```python
from build123d import *

# Parameters (mm, degrees)
CYLINDER099_R               = 3
CYLINDER099_DEPTH           = 3
CYLINDER098_R               = 5
CYLINDER098_DEPTH           = 3
CYLINDER090_R               = 1.2
CYLINDER090_DEPTH           = 13
CYLINDER091_R               = 1
CYLINDER091_DEPTH           = 12
CYLINDER091_ROLL_ANGLE      = 89.999919
CYLINDER091_PITCH_ANGLE     = -3.6e-05
CYLINDER091_PLACEMENT_ANGLE = 179.999964
CYLINDER069_R               = 2.2
CYLINDER069_DEPTH           = 12
CYLINDER069_ROLL_ANGLE      = 89.999919
CYLINDER069_PITCH_ANGLE     = -3.6e-05
CYLINDER069_PLACEMENT_ANGLE = 179.999964
CYLINDER068_R               = 1.2
CYLINDER068_DEPTH           = 12
CYLINDER068_ROLL_ANGLE      = 89.999919
CYLINDER068_PITCH_ANGLE     = -3.6e-05
CYLINDER068_PLACEMENT_ANGLE = 179.999964
BOX406016_W                 = 49
BOX406016_H                 = 2
BOX406016_DEPTH             = 32
BOX406008016_W              = 9
BOX406008016_H              = 12
BOX406008016_DEPTH          = 15
BOX406017_W                 = 16
BOX406017_H                 = 10.5
BOX406017_DEPTH             = 28
CYLINDER067_R               = 7
CYLINDER067_DEPTH           = 26
COMMON004_PLACEMENT_ANGLE   = 90
BOX406008015_W              = 15
BOX406008015_H              = 31
BOX406008015_DEPTH          = 15
BOX406008017_W              = 15
BOX406008017_H              = 4
BOX406008017_DEPTH          = 24
CYLINDER096_R               = 1.7
CYLINDER096_DEPTH           = 21
BOX_W                       = 15
BOX_H                       = 3
BOX_DEPTH                   = 8
CYLINDER097_R               = 1.7
CYLINDER097_DEPTH           = 21
BOX406008018_W              = 15
BOX406008018_H              = 3
BOX406008018_DEPTH          = 8
CHAMFER005_SIZE             = 1
CYLINDER093_R               = 1.7
CYLINDER093_DEPTH           = 21
CYLINDER092_R               = 1.7
CYLINDER092_DEPTH           = 21
BOX406008014_W              = 15
BOX406008014_H              = 3
BOX406008014_DEPTH          = 63
CHAMFER006_SIZE             = 1
CHAMFER007_SIZE             = 6.5
CHAMFER009_SIZE             = 0.5
CHAMFER010_SIZE             = 0.5


with BuildPart() as cylinder099:
    # Cylinder099 → Cylinder099 (new body)
    with BuildSketch(Plane(origin=(-9, -9, 36), x_dir=(1, 0, 0), z_dir=(0, 0, 1))):
        Circle(CYLINDER099_R)
    extrude(amount=CYLINDER099_DEPTH)


with BuildPart() as cut081:
    # Cylinder098 → Cylinder098 (new body)
    with BuildSketch(Plane(origin=(-9, -9, 36), x_dir=(1, 0, 0), z_dir=(0, 0, 1))):
        Circle(CYLINDER098_R)
    extrude(amount=CYLINDER098_DEPTH)

    # Cut081: cut Cylinder099
    add(cylinder099.part, mode=Mode.SUBTRACT)


with BuildPart() as cylinder084:
    # Cylinder090 → Cylinder090 (new body)
    with BuildSketch(Plane(origin=(0, 16, 35.8), x_dir=(1, 0, 0), z_dir=(0, -1, 0))):
        Circle(CYLINDER090_R)
    extrude(amount=CYLINDER090_DEPTH)


with BuildPart() as cylinder091:
    # Cylinder091 → Cylinder091 (new body)
    with BuildSketch(Plane.XY):
        Circle(CYLINDER091_R)
    extrude(amount=CYLINDER091_DEPTH)


with BuildPart() as cylinder091_1:
    # Cylinder091 roll: moved
    add(cylinder091.part.rotate(Axis((0, 0, 0), (1, 0, 0)), CYLINDER091_ROLL_ANGLE))


with BuildPart() as cylinder091_2:
    # Cylinder091 pitch: moved
    add(cylinder091_1.part.rotate(Axis((0, 0, 0), (0, 1, 0)), CYLINDER091_PITCH_ANGLE))


with BuildPart() as cylinder091_3:
    # Cylinder091 placement: moved
    add(cylinder091_2.part.moved(Location((11.75, -12, 42.5))).rotate(Axis((11.75, -12, 42.5), (0, 0, 1)), CYLINDER091_PLACEMENT_ANGLE))


with BuildPart() as cylinder069:
    # Cylinder069 → Cylinder069 (new body)
    with BuildSketch(Plane.XY):
        Circle(CYLINDER069_R)
    extrude(amount=CYLINDER069_DEPTH)


with BuildPart() as cylinder069_1:
    # Cylinder069 roll: moved
    add(cylinder069.part.rotate(Axis((0, 0, 0), (1, 0, 0)), CYLINDER069_ROLL_ANGLE))


with BuildPart() as cylinder069_2:
    # Cylinder069 pitch: moved
    add(cylinder069_1.part.rotate(Axis((0, 0, 0), (0, 1, 0)), CYLINDER069_PITCH_ANGLE))


with BuildPart() as cylinder069_3:
    # Cylinder069 placement: moved
    add(cylinder069_2.part.moved(Location((11.75, 3, 42.5))).rotate(Axis((11.75, 3, 42.5), (0, 0, 1)), CYLINDER069_PLACEMENT_ANGLE))


with BuildPart() as fusion103077013004017011:
    # Cylinder068 → Cylinder068 (new body)
    with BuildSketch(Plane.XY):
        Circle(CYLINDER068_R)
    extrude(amount=CYLINDER068_DEPTH)


with BuildPart() as fusion103077013004017011_1:
    # Cylinder068 roll: moved
    add(fusion103077013004017011.part.rotate(Axis((0, 0, 0), (1, 0, 0)), CYLINDER068_ROLL_ANGLE))


with BuildPart() as fusion103077013004017011_2:
    # Cylinder068 pitch: moved
    add(fusion103077013004017011_1.part.rotate(Axis((0, 0, 0), (0, 1, 0)), CYLINDER068_PITCH_ANGLE))


with BuildPart() as fusion103077013004017011_3:
    # Cylinder068 placement: moved
    add(fusion103077013004017011_2.part.moved(Location((11.75, 0, 42.5))).rotate(Axis((11.75, 0, 42.5), (0, 0, 1)), CYLINDER068_PLACEMENT_ANGLE))

    # Fusion103077013: union Cylinder069
    add(cylinder069_3.part)

    # Fusion103077013004017011: union Cylinder091
    add(cylinder091_3.part)


with BuildPart() as clamp_slot:
    # Box406016 → Box406016 (new body)
    with BuildSketch(Plane(origin=(48.48, 1, 22), x_dir=(-1, 0, 0), z_dir=(0, 0, 1))):
        with Locations((24.5, 1)):
            Rectangle(BOX406016_W, BOX406016_H)
    extrude(amount=BOX406016_DEPTH)


with BuildPart() as cube351:
    # Box406008016 → Box406008016 (new body)
    with BuildSketch(Plane(origin=(7, -6, 35), x_dir=(1, 0, 0), z_dir=(0, 0, 1))):
        with Locations((4.5, 6)):
            Rectangle(BOX406008016_W, BOX406008016_H)
    extrude(amount=BOX406008016_DEPTH)


with BuildPart() as gearbox001:
    # Box406017 → Box406017 (new body)
    with BuildSketch(Plane(origin=(-8, -5.25, 18), x_dir=(1, 0, 0), z_dir=(0, 0, 1))):
        with Locations((8, 5.25)):
            Rectangle(BOX406017_W, BOX406017_H)
    extrude(amount=BOX406017_DEPTH)


with BuildPart() as motor_hole:
    # Cylinder067 → Cylinder067 (new body)
    with BuildSketch(Plane.XY.offset(20)):
        Circle(CYLINDER067_R)
    extrude(amount=CYLINDER067_DEPTH)

    # Common004: intersect gearbox001
    add(gearbox001.part, mode=Mode.INTERSECT)


with BuildPart() as motor_hole_1:
    # Common004 placement: moved
    add(motor_hole.part.moved(Location((0, 0, 5))).rotate(Axis((0, 0, 5), (0, 0, 1)), COMMON004_PLACEMENT_ANGLE))


with BuildPart() as cut075:
    # Box406008015 → Box406008015 (new body)
    with BuildSketch(Plane(origin=(-7.5, -22, 35), x_dir=(1, 0, 0), z_dir=(0, 0, 1))):
        with Locations((7.5, 15.5)):
            Rectangle(BOX406008015_W, BOX406008015_H)
    extrude(amount=BOX406008015_DEPTH)

    # Cut073: cut motor-hole
    add(motor_hole_1.part, mode=Mode.SUBTRACT)

    # Fusion103077013004017010: union Cube351
    add(cube351.part)

    # Cut074: cut clamp-slot
    add(clamp_slot.part, mode=Mode.SUBTRACT)

    # Cut075: cut Fusion103077013004017011
    add(fusion103077013004017011_3.part, mode=Mode.SUBTRACT)


with BuildPart() as cut082:
    # Box406008017 → Box406008017 (new body)
    with BuildSketch(Plane(origin=(-7.5, 7, 26), x_dir=(1, 0, 0), z_dir=(0, 0, 1))):
        with Locations((7.5, 2)):
            Rectangle(BOX406008017_W, BOX406008017_H)
    extrude(amount=BOX406008017_DEPTH)

    # Fusion103077013004017012: union Cut075
    add(cut075.part)

    # Cut076: cut Cylinder084
    add(cylinder084.part, mode=Mode.SUBTRACT)


with BuildPart() as cut082_1:
    # Cut076 placement: moved
    add(cut082.part.moved(Location((0, 0, -5))))

    # Cut082: cut Cut081
    add(cut081.part, mode=Mode.SUBTRACT)


with BuildPart() as cylinder096:
    # Cylinder096 → Cylinder096 (new body)
    with BuildSketch(Plane(origin=(0, -13, 49), x_dir=(1, 0, 0), z_dir=(0, -1, 0))):
        Circle(CYLINDER096_R)
    extrude(amount=CYLINDER096_DEPTH)


with BuildPart() as cut080:
    # Box → Box (new body)
    with BuildSketch(Plane(origin=(-7.5, -25, 45), x_dir=(1, 0, 0), z_dir=(0, 0, 1))):
        with Locations((7.5, 1.5)):
            Rectangle(BOX_W, BOX_H)
    extrude(amount=BOX_DEPTH)

    # Cut080: cut Cylinder096
    add(cylinder096.part, mode=Mode.SUBTRACT)


with BuildPart() as cylinder097:
    # Cylinder097 → Cylinder097 (new body)
    with BuildSketch(Plane(origin=(0, -13, -22), x_dir=(1, 0, 0), z_dir=(0, -1, 0))):
        Circle(CYLINDER097_R)
    extrude(amount=CYLINDER097_DEPTH)


with BuildPart() as chamfer005:
    # Box406008018 → Box406008018 (new body)
    with BuildSketch(Plane(origin=(-7.5, -25, -26), x_dir=(1, 0, 0), z_dir=(0, 0, 1))):
        with Locations((7.5, 1.5)):
            Rectangle(BOX406008018_W, BOX406008018_H)
    extrude(amount=BOX406008018_DEPTH)

    # Cut079: cut Cylinder097
    add(cylinder097.part, mode=Mode.SUBTRACT)

    # Fusion103077013004017015: union Cut080
    add(cut080.part)

    # Chamfer005
    chamfer005_edges = [chamfer005.edges().sort_by_distance(p)[0] for p in [
        (-1.7, -22, -22),
        (-1.7, -22, 49),
    ]]
    chamfer(chamfer005_edges, length=CHAMFER005_SIZE)


with BuildPart() as cylinder093:
    # Cylinder093 → Cylinder093 (new body)
    with BuildSketch(Plane(origin=(3, -13, -4), x_dir=(1, 0, 0), z_dir=(0, -1, 0))):
        Circle(CYLINDER093_R)
    extrude(amount=CYLINDER093_DEPTH)


with BuildPart() as fusion103077013004017013:
    # Cylinder092 → Cylinder092 (new body)
    with BuildSketch(Plane(origin=(-3, -13, -14), x_dir=(1, 0, 0), z_dir=(0, -1, 0))):
        Circle(CYLINDER092_R)
    extrude(amount=CYLINDER092_DEPTH)

    # Fusion103077013004017013: union Cylinder093
    add(cylinder093.part)


with BuildPart() as chamfer010:
    # Box406008014 → Box406008014 (new body)
    with BuildSketch(Plane(origin=(-7.5, -25, -18), x_dir=(1, 0, 0), z_dir=(0, 0, 1))):
        with Locations((7.5, 1.5)):
            Rectangle(BOX406008014_W, BOX406008014_H)
    extrude(amount=BOX406008014_DEPTH)

    # Cut077: cut Fusion103077013004017013
    add(fusion103077013004017013.part, mode=Mode.SUBTRACT)

    # Chamfer006
    chamfer006_edges = [chamfer010.edges().sort_by_distance(p)[0] for p in [
        (-4.7, -25, -14),
        (1.3, -25, -4),
    ]]
    chamfer(chamfer006_edges, length=CHAMFER006_SIZE)

    # Fusion103077013004017016: union Chamfer005
    add(chamfer005.part)

    # Chamfer007
    chamfer007_edges = [chamfer010.edges().sort_by_distance(p)[0] for p in [
        (-7.5, -23.5, -26),
        (7.5, -23.5, -26),
        (7.5, -23.5, 53),
        (-7.5, -23.5, 53),
    ]]
    chamfer(chamfer007_edges, length=CHAMFER007_SIZE)

    # Fusion103077013004017017: union Cut082
    add(cut082_1.part)

    # Chamfer009
    chamfer009_edges = [chamfer010.edges().sort_by_distance(p)[0] for p in [
        (-4.7, -22, -14),
        (1.3, -22, -4),
    ]]
    chamfer(chamfer009_edges, length=CHAMFER009_SIZE)

    # Chamfer010
    chamfer010_edges = [chamfer010.edges().sort_by_distance(p)[0] for p in [
        (-1.7, -25, -22),
        (-1.7, -25, 49),
    ]]
    chamfer(chamfer010_edges, length=CHAMFER010_SIZE)


solid = chamfer010.part
```
The model under review builds one solid part; all positions refer to its coordinate system, in mm. A direction names the side the tool comes from. Coordinates: 2 decimals unless noted, no trailing zeros. Write each loop counter-clockwise with the first axis right and the second up, starting at its lowest first coordinate (ties: lowest second). Pieces come first, ordered by that corner, then holes. Notation, with made-up numbers: (7.25, 33) -> (59.25, 33) arc R14 ccw to (59.25, 42) -> close; hole circle Ø9 at (21.25, 53). An arc over 180 degrees is marked (long way). One line per item, written item: value. Start each with the question number.
Q1. Add section A-A, the plane z = -14. Give the boundary of the cut face in (x, y), then the cut area to 4 significant figures.
Q2. Clearance check with flat-ended pins moving along their axes: P1, Ø2.5, axis at x = 0, z = 49, coming from the +Y side; P2, Ø1.8, axis at x = -6.5, y = -7.5, coming from the +Z side; P3, Ø4, axis at y = -19.5, z = 44, coming from the +X side; P4, Ø6.5, axis at x = 5.5, y = 3.5, coming from the -Z side. State where each tip first meets the part, or that it passes through.
Q3. To check wall thickness, follow probe 1 along Z at (x, y) = (0, -24.05); probe 2 along X at (y, z) = (-3.45, 37.5); probe 3 along Z at (x, y) = (11.75, 5.15). State the ranges of each line that lie inside material, in increasing order.
Q4. The part is to be moulded in two halves that separate along Y. For faces 1 (the face through (-0.221, -23.74, -20.314)), 2 (the face through (0, -22, 46)), 3 (the face through (10, 4, 30)), 4 (the face through (0, 7, 25)), say which applies: +Y half, -Y half, draft (parallel to the pull), parting line (faces both ways), or undercut.
Q5. Add section D-D, the plane y = -12.5. Give the boundary of the cut face in (x, z).
Q6. Add section C-C, the plane z = 49. Give the boundary of the cut face in (x, y), then the cut area to 4 significant figures.
Q7. Add section B-B, the plane y = 2. Count the separate pieces of the cut face and the enclosed holes in it, then the cut area to 3 significant figures.
Q8. For faces 5 (the face through (5.25, -3, 37)), 6 (the face through (10, -1, 37)), 7 (the face through (0, -23, 53)), 8 (the face through (-0.26, 8.98, 29.63)), 9 (the face through (7.5, 8, 33)), list the 3-axis set-ups (+Z, -Z, +X, -X, +Y, -Y) from which the entire face can be reached by the end or side of a thin tool; tool diameter is ignored.
Response:
1. outline: (-7.5, -25) -> (-5.7, -25) -> (-4.7, -24) -> (-4.7, -22.5) -> (-5.2, -22) -> (-7.5, -22) -> close; (-1.3, -24) -> (-0.3, -25) -> (7.5, -25) -> (7.5, -22) -> (-0.8, -22) -> (-1.3, -22.5) -> close
1. area: 33.55 mm²
2. P1: through
2. P2: z = 45
2. P3: x = 7.5
2. P4: z = 30
3. probe 1: -26 to -23.7, -20.3 to 47.3, 50.7 to 53
3. probe 2: -7.5 to -5.25, 5.25 to 10.75, 12.75 to 16
3. probe 3: 30 to 35.3, 39.7 to 45
4. face 1: draft
4. face 2: +Y half
4. face 3: undercut
4. face 4: undercut
5. outline: (-7.5, 30) -> (7.5, 30) -> (7.5, 45) -> (-7.5, 45) -> (-7.5, 39) -> (-5.43, 39) -> (-5.43, 36) -> (-7.5, 36) -> close
6. outline: (-5, -25) -> (-2.2, -25) -> (-1.7, -24.5) -> (-1.7, -23) -> (-2.7, -22) -> (-5, -22) -> close; (1.7, -24.5) -> (2.2, -25) -> (5, -25) -> (5, -22) -> (2.7, -22) -> (1.7, -23) -> close
6. area: 18.55 mm²
7. separate pieces: 2
7. enclosed holes: 1
7. area: 190 mm²
8. face 5: +Z, -Z
8. face 6: +Z, -Z, +X
8. face 7: +Z, +X, -X, +Y, -Y
8. face 8: +Y
8. face 9: +Z, -Z, +X, +Y
